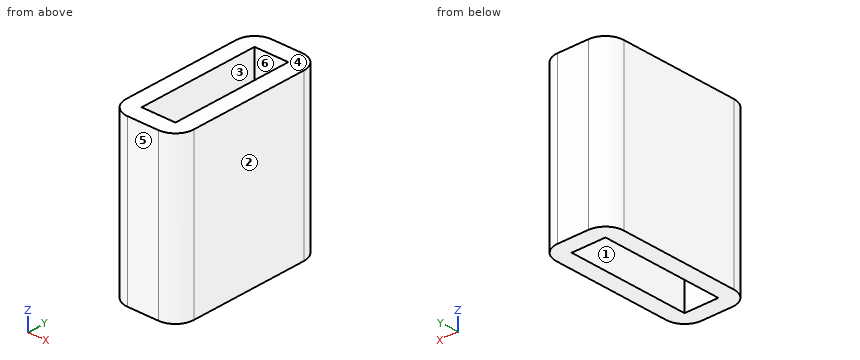
Autodesk Inventor part; units mm, degrees
ref_plane "YZ Plane" through (0, 0, 0) normal (1, 0, 0) x (0, 1, 0)
ref_plane "XZ Plane" through (0, 0, 0) normal (0, 1, 0) x (-1, 0, 0)
ref_plane "XY Plane" through (0, 0, 0) normal (0, 0, 1) x (1, 0, 0)
sketch "Sketch1" plane through (0, 0, 0) normal (0, 0, 1) x (1, 0, 0)
  line L0 (-1.1, 4) -> (1.1, 4)
  line L1 (1.1, 4) -> (1.1, -4)
  line L2 (1.1, -4) -> (-1.1, -4)
  line L3 (-1.1, -4) -> (-1.1, 4)
  line L4 (-2.2, 5.1) -> (2.2, 5.1)
  line L5 (2.2, 5.1) -> (2.2, -5.1)
  line L6 (2.2, -5.1) -> (-2.2, -5.1)
  line L7 (-2.2, -5.1) -> (-2.2, 5.1)
  point P0 (0, 0)
  dimension "d0" = 2.2
  dimension "d1" = 8
  dimension "d2" = 1.1
  dimension "d3" = 4
  dimension "d4" = 2.2
  dimension "d5" = 2.2
  dimension "d6" = 1.1
  dimension "d7" = 1.1
  dimension "d8" = 1.1
extrude "Extrusion1" add sketch "Sketch1" along normal blind 10.5
fillet "Fillet1" radius 1.2 4 edges at (2.2, 5.1, 5.25) (-2.2, 5.1, 5.25) (-2.2, -5.1, 5.25) (2.2, -5.1, 5.25)
equation "\"d7\" = d6"
equation "\"d8\" = d6"
properties part number "coil"
Design review of the part built by this model. Coordinates are the model's own, in mm. Face numbers are marked on the shaded views. A direction names the side the tool comes from. Give positions to 0.01 mm unless a question says otherwise; leave off trailing zeros. Order: outer loops, then holes, each group sorted by start corner. A loop starts at its lowest first (then second) coordinate and runs counter-clockwise, first axis right, second up. Notation, with made-up numbers: (-23.75, -10.5) -> (2.25, -10.5) arc R26 ccw to (2.25, 7.5) -> close; hole circle Ø9 at (26, 35.25). An arc over 180 degrees is marked (long way). Write each question's results on one line, items separated by ' | '. Start each with the question number.
Q1. Add section C-C on z = 1.25. Give the boundary of the cut face in (x, y).
Q2. Wall thickness on L1, parallel to X at y = -2.5, z = 6; L2, parallel to Y at x = 0.75, z = 2.75; L3, parallel to Y at x = -1.3, z = 6: over which ranges is each line inside the solid? List them lowest first. Write a range as from..to.
Q3. Mouldability with a two-part tool opening along Y and no side actions: class the marked faces 3, 4, 5 and 6 as +Y half, -Y half, draft (parallel to the pull), parting line (faces both ways), or undercut.
Q4. Machinability: for the marked faces 1 and 2, which of the approach directions +Z, -Z, +X, -X, +Y, -Y give a long, thin tool a straight path to every point of the face, cutting with its end or side? Answer none if there is none.
Q5. Add section B-B on y = 1. Give the boundary of the cut face in (x, z), and give its area (3 significant figures).
Q6. Add section A-A on x = 0.3. Give the boundary of the cut face in (y, z), and give its area (3 significant figures).
Found:
1) outline: (-2.2, -3.9) arc R1.2 ccw to (-1, -5.1) -> (1, -5.1) arc R1.2 ccw to (2.2, -3.9) -> (2.2, 3.9) arc R1.2 ccw to (1, 5.1) -> (-1, 5.1) arc R1.2 ccw to (-2.2, 3.9) -> close; hole (-1.1, -4) -> (1.1, -4) -> (1.1, 4) -> (-1.1, 4) -> close
2) L1: x = -2.2..-1.1, 1.1..2.2 | L2: y = -5.1..-4, 4..5.1 | L3: y = -5.06..5.06
3) face 3: undercut | face 4: draft | face 5: -Y half | face 6: undercut
4) face 1: +Z, -Z | face 2: +Z, -Z, +X, +Y, -Y
5) outline: (-2.2, 0) -> (-1.1, 0) -> (-1.1, 10.5) -> (-2.2, 10.5) -> close; (1.1, 0) -> (2.2, 0) -> (2.2, 10.5) -> (1.1, 10.5) -> close | area: 23.1 mm2
6) outline: (-5.1, 0) -> (-4, 0) -> (-4, 10.5) -> (-5.1, 10.5) -> close; (4, 0) -> (5.1, 0) -> (5.1, 10.5) -> (4, 10.5) -> close | area: 23.1 mm2
